Drawing for the job (mm, zero at the part's lowest x, y, z). A direction names the side the tool comes from. Coordinates: 2 decimals unless noted, no trailing zeros. Write each loop counter-clockwise with the first axis right and the second up, starting at its lowest first coordinate (ties: lowest second). Pieces come first, ordered by that corner, then holes. Notation, with made-up numbers: M 50.25,13 L 81.25,13 A10 cw 81.25,22 Z; hole C 51.25,22.25 d4. An arc over 180 degrees is marked long. Put each result on its own line as item: value. Start each with the question number.
Q1. Cut at B-B (y = 12). Write the cut outline in (x, z).
Q2. Drill centre lines: line 1 along Y through (x, z) = (11, 7.5); line 2 along Y through (x, z) = (6, 4); line 3 along X through (y, z) = (31, 5) (1 decimal). Where is each one in solid material? Low to high.
Q3. Which spindle directions (+Z, -Z, +X, -X, +Y, -Y) get a long thin tool onto all of the face, cutting with end or side? Do the marked faces 4, 5 and 6. Say none if no direction does.
Q4. Drop flat-ended pins along their axis: pin 1 (2.5 mm diameter, centred on x = 7.5, z = 6, fed in from +Y); pin 2 (5 mm diameter, centred on y = 23.5, z = 4, fed in from +X); pin 3 (6 mm diameter, centred on y = 22.5, z = 1.5, fed in from +X) (1 decimal). Give the stop position or say it passes through.
Q5. Pull direction X, two halves, no side cores. Call the marked faces 1, 2 and 3: pulls with the +X half, pulls with the -X half, needs draft (parallel to the pull), parting line crosses it, or undercut.
Q6. Cut at A-A (z = 6.5). Write the cut outline in (x, y).
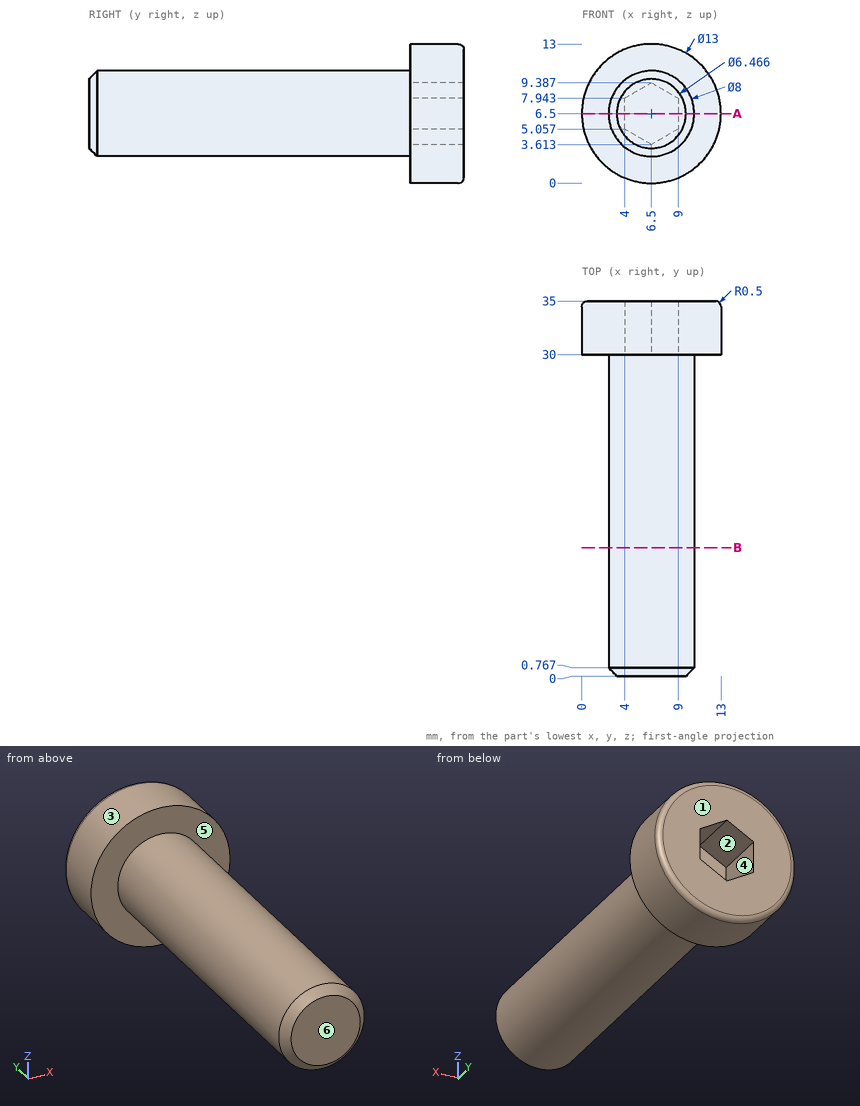
Computed values:
1. outline: C 6.5,6.5 d8
2. line 1: 30 to 35
2. line 2: 0 to 30
2. line 3: 0.2 to 4.1, 8.9 to 12.8
3. face 4: +Y
3. face 5: -Y
3. face 6: +Z, -Z, +X, -X, -Y
4. pin 1: y = 30
4. pin 2: x = 10.5
4. pin 3: x = 10
5. face 1: needs draft
5. face 2: undercut
5. face 3: parting line crosses it
6. outline: M 0,30 L 2.5,30 L 2.5,0.77 L 3.27,0 L 9.73,0 L 10.5,0.77 L 10.5,30 L 13,30 L 13,34.5 A0.5 ccw 12.5,35 L 9,35 L 9,30 L 4,30 L 4,35 L 0.5,35 A0.5 ccw 0,34.5 Z
